Here's how the part is built. I have some questions about the finished solid (model axes, mm). A direction names the side the tool comes from. Round coordinates to 2 decimals unless told otherwise and drop trailing zeros. Order: outer loops, then holes, each group sorted by start corner. A loop starts at its lowest first (then second) coordinate and runs counter-clockwise, first axis right, second up. Notation, with made-up numbers: (-37, 56) -> (-33, 56) arc R33 ccw to (-33, 84) -> close; hole circle Ø1 at (65.5, -37). An arc over 180 degrees is marked (long way). One line per item, written item: value.
```python
from build123d import *

# Parameters (mm, degrees)
F0_W     = 1047.75
F0_H     = 342.9
F1_DEPTH = 38.1
F2_R     = 38.1
F3_W     = 25.4
F3_H     = 85.725
F4_DEPTH = 50.8


with BuildPart() as f1:
    # F0 (on Top) → F1 (new body)
    with BuildSketch(Plane.XY):
        Rectangle(F0_W, F0_H)
    extrude(amount=F1_DEPTH)

    # F2
    f2_edges = [f1.edges().sort_by_distance(p)[0] for p in [
        (-523.875, 171.45, 19.05),
        (-523.875, -171.45, 19.05),
        (523.875, 171.45, 19.05),
        (523.875, -171.45, 19.05),
    ]]
    fillet(f2_edges, radius=F2_R)

    # F3 (on face) → F4 (cut)
    with BuildSketch(Plane.XY.offset(38.1)):
        with Locations((511.175, 128.5875)):
            Rectangle(F3_W, F3_H)
        with Locations((511.175, -128.5875)):
            Rectangle(F3_W, F3_H)
    extrude(amount=-F4_DEPTH, mode=Mode.SUBTRACT)


solid = f1.part
```
Q1. I need wall thicknesses on line 1 along X through (y, z) = (98, 6.5) (3 decimals). Which ranges of the line are inside material? Lowest first, please.
Answers:
line 1: -523.875 to 498.475
Q2. I want a section at B-B on y = 145. Write out the boundary of the cut face in (x, z) (3 decimals), then the cut area to 3 significant figures.
Answers:
outline: (-522.05, 0) -> (498.475, 0) -> (498.475, 38.1) -> (-522.05, 38.1) -> close
area: 38,900 mm2
Q3. I want a section at A-A on y = -95. Write out the boundary of the cut face in (x, z) (3 decimals), then the cut area to 3 significant figures.
Answers:
outline: (-523.875, 0) -> (498.475, 0) -> (498.475, 38.1) -> (-523.875, 38.1) -> close
area: 39,000 mm2
Q4. Which directions (+Z, -Z, +X, -X, +Y, -Y) give clear straight access to the entire face, cutting with the end or side of a thin tool? Please do faces 1 (the face through (511, -85.725, 19)), 2 (the face through (-523.875, -2, 19)), 3 (the face through (511, 85.725, 19)).
Answers:
face 1: +Z, -Z, +X, -Y
face 2: +Z, -Z, -X, +Y, -Y
face 3: +Z, -Z, +X, +Y
Q5. For P1, Ø4, axis at y = -136.5, z = 26, coming from the +X side (3 decimals); P2, Ø7.5, axis at x = 508.5, z = 22, coming from the +Y side (3 decimals); P3, Ø20.5, axis at x = 510.5, z = 26.5, coming from the -Y side (3 decimals), each with a flat end and sliding along its axis, tell me the tip position at first contact or that it passes through.
Answers:
P1: x = 498.475
P2: y = 85.725
P3: y = -85.725
